```python
from build123d import *

# Parameters (mm, degrees)
SKETCH_1_R      = 1.25
EXTRUDE_1_DEPTH = 1.6


with BuildPart() as part:
    # Эскиз1 → Бобышка-Вытянуть1 (new body)
    with BuildSketch(Plane(origin=(0, 0, 0), x_dir=(1, 0, 0), z_dir=(0, 1, 0))):
        Polygon((-32, -24), (-32, 22), (-31, 23), (-17, 23), (-16, 24), (-16, 29), (-15, 30), (-6, 30), (-5, 31), (-5, 34), (-3, 36), (3, 36), (5, 34), (5, 31), (6, 30), (26, 30), (31, 25), (31, -22), (18, -35), (15, -35), (13, -37), (-8, -37), (-9, -36), (-9, -33), (-10, -32), (-24, -32), align=None)
        with Locations(Location((-25, -24, 0), (0, 0, 270))):
            Circle(SKETCH_1_R, mode=Mode.SUBTRACT)
        with Locations(Location((25, -24, 0), (0, 0, 90))):
            Circle(SKETCH_1_R, mode=Mode.SUBTRACT)
        with Locations(Location((0, 32, 0), (0, 0, 270))):
            Circle(SKETCH_1_R, mode=Mode.SUBTRACT)
        with Locations(Location((-12, -10, 0), (0, 0, 270))):
            Circle(SKETCH_1_R, mode=Mode.SUBTRACT)
        with Locations(Location((-12, 10, 0), (0, 0, 90))):
            Circle(SKETCH_1_R, mode=Mode.SUBTRACT)
    extrude(amount=EXTRUDE_1_DEPTH)


solid = part.part
```
Work out the finished part from the listing and answer in its coordinate system (mm). A direction names the side the tool comes from. Give positions to 0.01 mm unless a question says otherwise; leave off trailing zeros. Loops run counter-clockwise (first coordinate to the right, second up) from the corner with the lowest first, then second, coordinate; pieces in that order, holes last. Notation, with made-up numbers: M 36.5,16 L 42.5,16 A21 ccw 42.5,32 Z; hole C -26.75,11 d5. An arc over 180 degrees is marked long. One line per item, written item: value. Start each with the question number.
1. Find section A-A (x = 25). Give the vertices of the cut face in (y, z), and give its area (3 significant figures).
2. Find the intervals of material crossed by probe 1 along X at (y, z) = (0.8, 10); probe 2 along X at (y, z) = (0.8, -32); probe 3 along Z at (x, y) = (-22.5, 1.55), in increasing order.
3. Which of the six approach directions +Z, -Z, +X, -X, +Y, -Y give full straight-line access (tool end or side, diameter ignored) to faces 4 (the face through (0, 0, 0)), 5 (the face through (-0.479, 0.789, -30.845)), 6 (the face through (-9, 1, 35)), 7 (the face through (17, 1, 35)), 8 (the face through (-11, 1, -30))?
4. Find section C-C (y = 1). State how many separate pieces and enclosed holes the cut face has, and give its area (3 significant figures).
5. Each of these flat-tipped pins is pushed along its axis until it touches: P1, Ø0.5, axis at x = 19.5, y = 1, coming from the -Z side; P2, Ø0.5, axis at x = -20, y = 1, coming from the +Z side; P3, Ø0.5, axis at y = 1, z = -27, coming from the -X side; P4, Ø1.5, axis at x = -12, z = -10, coming from the +Y side. Where does it stop, or does it pass through?
6. Find section D-D (x = -12). Give the vertices of the cut face in (y, z), and give its area (3 significant figures).
7. Find section B-B (z = -10). Give the vertices of the cut face in (x, y), and give its area (3 significant figures).
8. Determine the mould class of faces 1 (the face through (-5, 1, -32)), 2 (the face through (5, 1, -33)), 3 (the face through (-12.845, 0.789, -9.079)) for opening direction X: released by +X, released by -X, zero draft, split by the parting line, or undercut.
Reported:
1. outline: M 0,-30 L 1.6,-30 L 1.6,22.75 L 0,22.75 Z; M 0,25.25 L 1.6,25.25 L 1.6,28 L 0,28 Z
1. area: 88.8 mm²
2. probe 1: x = -32 to -13.25, -10.75 to 31
2. probe 2: x = -5 to -1.25, 1.25 to 5
2. probe 3: z = -23 to 32
3. face 4: +Z, -Z, +X, -X, -Y
3. face 5: +Y, -Y
3. face 6: +Z, -X, +Y, -Y
3. face 7: +Z, +X, +Y, -Y
3. face 8: -Z, -X, +Y, -Y
4. separate pieces: 1
4. enclosed holes: 5
4. area: 3,860 mm²
5. P1: stops at z = -30
5. P2: stops at z = 32
5. P3: stops at x = -16
5. P4: passes through
6. outline: M 0,-30 L 1.6,-30 L 1.6,-11.25 L 0,-11.25 Z; M 0,-8.75 L 1.6,-8.75 L 1.6,8.75 L 0,8.75 Z; M 0,11.25 L 1.6,11.25 L 1.6,32 L 0,32 Z
6. area: 91.2 mm²
7. outline: M -32,0 L -13.25,0 L -13.25,1.6 L -32,1.6 Z; M -10.75,0 L 31,0 L 31,1.6 L -10.75,1.6 Z
7. area: 96.8 mm²
8. face 1: released by -X
8. face 2: released by +X
8. face 3: undercut
